```python
from build123d import *

# Parameters (mm, degrees)
SKETCH_1_W      = 42.04
SKETCH_1_H      = 27.22
EXTRUDE_1_DEPTH = 1.4
SKETCH_2_W      = 37.052
SKETCH_2_H      = 19.516
EXTRUDE_2_DEPTH = 0.1
SKETCH_3_W      = 12.5
SKETCH_3_H      = 0.3
EXTRUDE_3_DEPTH = 36.1


with BuildPart() as part:
    # 草图1 → 凸台-拉伸1 (new body)
    with BuildSketch(Plane(origin=(0, 0, 0), x_dir=(1, 0, 0), z_dir=(0, 1, 0))):
        Rectangle(SKETCH_1_W, SKETCH_1_H)
    extrude(amount=EXTRUDE_1_DEPTH)

    # 草图2 → 凸台-拉伸2 (add)
    with BuildSketch(Plane(origin=(0, 1.4, 0), x_dir=(1, 0, 0), z_dir=(0, 1, 0))):
        with Locations((0, 1.852)):
            Rectangle(SKETCH_2_W, SKETCH_2_H)
    extrude(amount=EXTRUDE_2_DEPTH)

    # 草图3 → 凸台-拉伸3 (add)
    with BuildSketch(Plane.XY.offset(13.61)):
        with Locations((0, 1.031860601)):
            Rectangle(SKETCH_3_W, SKETCH_3_H)
    extrude(amount=EXTRUDE_3_DEPTH)


solid = part.part
```
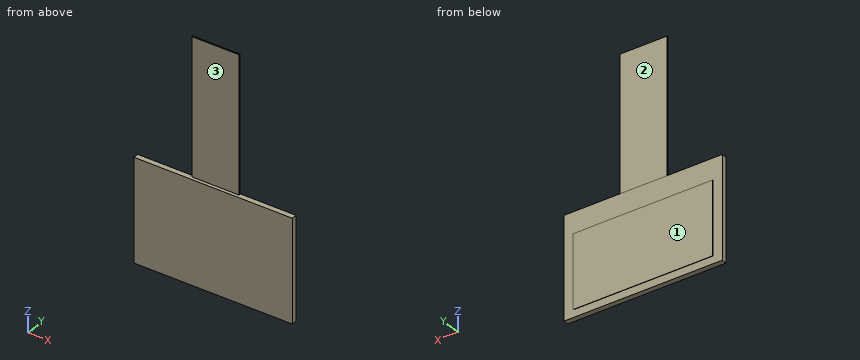
Check sheet for the modelled part. Datum: model origin and axes. Units: mm. Face numbers are marked on the shaded views. A direction names the side the tool comes from. Round coordinates to 2 decimals unless told otherwise and drop trailing zeros. Order: outer loops, then holes, each group sorted by start corner. A loop starts at its lowest first (then second) coordinate and runs counter-clockwise, first axis right, second up.
1) Section check B-B (y = 0.6). Record the boundary of the cut face in (x, z), and give its area (3 significant figures).
2) Section check C-C (z = 28). Record the boundary of the cut face in (x, y), and give its area (3 significant figures).
3) Section check D-D (x = 10.5). Record the boundary of the cut face in (y, z).
4) Go/stop test with flat-tipped pins: pin 1 Ø10 at (x, z) = (6, 39) entering from -Y; pin 2 Ø12 at (x, z) = (13, 32) entering from +Y; pin 3 Ø6 at (x, z) = (1, 30) entering from +Y; pin 4 Ø0.7 at (x, y) = (10, 1) entering from +Z. Record where each tip stops, or that it passes through.
5) Section check A-A (x = 3.5). Record the boundary of the cut face in (y, z), and give its area (3 significant figures).
6) Scan line: line 1 (Z direction, x = -2.5, y = 0.4). Record every from-to range of solid material in increasing order.
7) Tool access check on the marked faces 1, 2 and 3. Record the directions out of +Z, -Z, +X, -X, +Y, -Y that give a thin tool (end or side, any length) a straight path to the whole face; none if there is none.
Result:
1. outline: (-21.02, -13.61) - (21.02, -13.61) - (21.02, 13.61) - (-21.02, 13.61) - close
1. area: 1,140 mm2
2. outline: (-6.25, 0.88) - (6.25, 0.88) - (6.25, 1.18) - (-6.25, 1.18) - close
2. area: 3.75 mm2
3. outline: (0, -13.61) - (1.4, -13.61) - (1.4, -11.61) - (1.5, -11.61) - (1.5, 7.91) - (1.4, 7.91) - (1.4, 13.61) - (0, 13.61) - close
4. pin 1: stops at y = 0.88
4. pin 2: passes through
4. pin 3: stops at y = 1.18
4. pin 4: stops at z = 13.61
5. outline: (0, -13.61) - (1.4, -13.61) - (1.4, -11.61) - (1.5, -11.61) - (1.5, 7.91) - (1.4, 7.91) - (1.4, 13.61) - (1.18, 13.61) - (1.18, 49.71) - (0.88, 49.71) - (0.88, 13.61) - (0, 13.61) - close
5. area: 50.9 mm2
6. line 1: z = -13.61 to 13.61
7. face 1: +Z, -Z, +X, -X, +Y
7. face 2: +Z, +X, -X, +Y
7. face 3: +Z, +X, -X, -Y
